Part print with two shaded views. Sizes in mm from the minimum x, y, z corner. A direction names the side the tool comes from. Give positions to 0.01 mm unless a question says otherwise; leave off trailing zeros. Write each loop counter-clockwise with the first axis right and the second up, starting at its lowest first coordinate (ties: lowest second). Pieces come first, ordered by that corner, then holes.
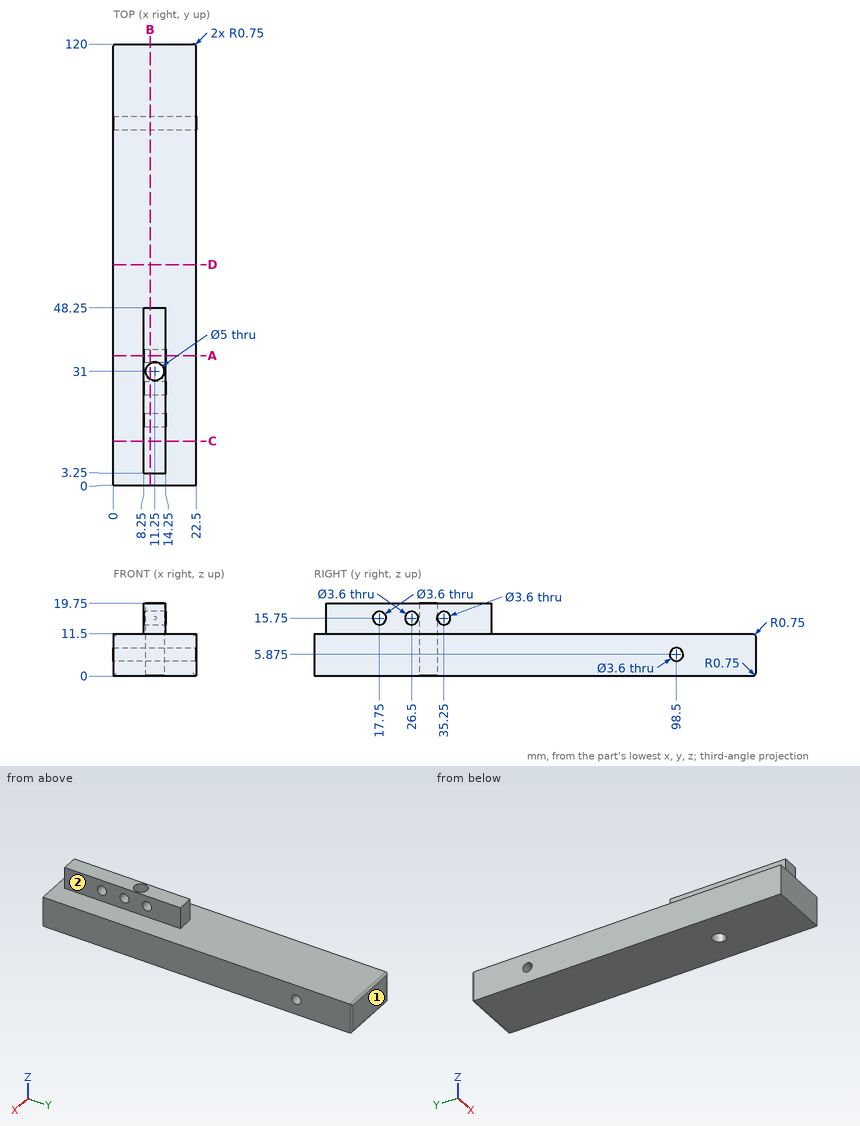
(1) Saw through at C-C, the plane y = 12. List the corners of the cut face in (x, z), plus the area to 3 significant figures.
(2) Drop flat-ended pins along their axis: pin 1 (3 mm diameter, centred on y = 17.75, z = 15.75, fed in from +X); pin 2 (4.5 mm diameter, centred on y = 26.5, z = 15.75, fed in from +X); pin 3 (1.8 mm diameter, centred on x = 12.5, z = 17, fed in from -Y); pin 4 (12 mm diameter, centred on x = 3, y = 69.5, fed in from +Z). Give the stop position or say it passes through.
(3) Saw through at B-B, the plane x = 10. List the corners of the cut face in (y, z) (3 decimals), plus the area to 3 significant figures.
(4) Probe line 1 (Y direction, x = 11.5, z = 15.75); line 2 (Z direction, x = 9.65, y = 26.5); line 3 (Y direction, x = 10, z = 15.75). List the from-to ranges inside material, lowest first.
(5) 3-axis set-ups, long thin cutter, end or side, ignore diameter. For the marked faces 1 and 2: which of +Z, -Z, +X, -X, +Y, -Y reach the whole face in a straight line?
(6) Saw through at A-A, the plane y = 35.25. List the corners of the cut face in (x, z), plus the area to 3 significant figures.
(7) Saw through at D-D, the plane y = 60. List the corners of the cut face in (x, z).
Computed values:
1. outline: (0, 0) - (22.5, 0) - (22.5, 11.5) - (14.25, 11.5) - (14.25, 19.75) - (8.25, 19.75) - (8.25, 11.5) - (0, 11.5) - close
1. area: 308 mm2
2. pin 1: passes through
2. pin 2: stops at x = 14.25
2. pin 3: stops at y = 3.25
2. pin 4: stops at z = 11.5
3. outline: (0, 0) - (28.835, 0) - (28.835, 19.75) - (3.25, 19.75) - (3.25, 11.5) - (0, 11.5) - close; (33.165, 0) - (119.25, 0) arc R0.75 ccw to (120, 0.75) - (120, 10.75) arc R0.75 ccw to (119.25, 11.5) - (48.25, 11.5) - (48.25, 19.75) - (33.165, 19.75) - close; hole circle Ø3.6 at (17.75, 15.75); hole circle Ø3.6 at (26.5, 15.75); hole circle Ø3.6 at (35.25, 15.75); hole circle Ø3.6 at (98.5, 5.875)
3. area: 1,620 mm2
4. line 1: y = 3.25 to 15.95, 19.55 to 24.7, 28.3 to 28.51, 37.05 to 48.25
4. line 2: z = 0 to 13.95, 17.55 to 19.75
4. line 3: y = 3.25 to 15.95, 19.55 to 24.7, 28.3 to 28.83, 33.17 to 33.45, 37.05 to 48.25
5. face 1: +Z, -Z, +X, -X, +Y
5. face 2: +Z, +X, +Y, -Y
6. outline: (0, 0) - (22.5, 0) - (22.5, 11.5) - (14.25, 11.5) - (14.25, 13.95) - (8.25, 13.95) - (8.25, 11.5) - (0, 11.5) - close; (8.25, 17.55) - (14.25, 17.55) - (14.25, 19.75) - (8.25, 19.75) - close
6. area: 287 mm2
7. outline: (0, 0) - (22.5, 0) - (22.5, 11.5) - (0, 11.5) - close
